```python
from build123d import *

# Parameters (mm, degrees)
F0_R     = 12.5
F1_DEPTH = 3.175
F3_DEPTH = 25.4
F4_R     = 1.5
F5_DEPTH = 25


with BuildPart() as f1:
    # F0 (on Top) → F1 (new body)
    with BuildSketch(Plane.XY):
        with BuildLine():
            Line((61, 42.8), (-61, 42.8))
            ThreePointArc((-61, 42.8), (-63.12132, 41.92132), (-64, 39.8))
            Line((-64, 39.8), (-64, -39.8))
            ThreePointArc((-64, -39.8), (-63.12132, -41.92132), (-61, -42.8))
            Line((-61, -42.8), (61, -42.8))
            ThreePointArc((61, -42.8), (63.12132, -41.92132), (64, -39.8))
            Line((64, -39.8), (64, 39.8))
            ThreePointArc((64, 39.8), (63.12132, 41.92132), (61, 42.8))
        make_face()
        Circle(F0_R, mode=Mode.SUBTRACT)
    extrude(amount=F1_DEPTH)

    # F2 (on Top) → F3 (join)
    with BuildSketch(Plane.XY):
        with BuildLine():
            Line((-57.674601, -36.461943), (-64.024601, -36.461943))
            Line((-64.024601, -36.461943), (-64.024601, -39.811943))
            ThreePointArc((-64.024601, -39.811943), (-63.145921, -41.933263), (-61.024601, -42.811943))
            Line((-61.024601, -42.811943), (-57.674601, -42.811943))
            Line((-57.674601, -42.811943), (-57.674601, -36.461943))
        make_face()
    extrude(amount=-F3_DEPTH)

    # F4 (on Top) → F5 (cut)
    with BuildSketch(Plane.XY):
        with Locations((-48.248243, 0)):
            Circle(F4_R)
        with Locations((48.708693, 0)):
            Circle(F4_R)
    extrude(amount=F5_DEPTH, mode=Mode.SUBTRACT)


solid = f1.part
```
Geometry check sheet. Reference: the model listing, model coordinates, mm. A direction names the side the tool comes from. Coordinates: 2 decimals unless noted, no trailing zeros. Loops run counter-clockwise (first coordinate to the right, second up) from the corner with the lowest first, then second, coordinate; pieces in that order, holes last. Notation, with made-up numbers: (80, 68.5) -> (128, 68.5) arc R17 cw to (128, 82.5) -> close; hole circle Ø4 at (33, 50.5). An arc over 180 degrees is marked (long way). Put each result on its own line as item: value.
1) Cross-section at D-D on x = 56.5. Record the boundary of the cut face in (y, z) (3 decimals), plus the area to 3 significant figures.
Result set:
outline: (-42.8, 0) -> (42.8, 0) -> (42.8, 3.175) -> (-42.8, 3.175) -> close
area: 272 mm^2
2) Release check for a two-part mould opening along Y. For faces 1 (the cylindrical face through (-49.747, 0.066, 1.565)), 2 (the flat face through (64, -1, 2)), 3 (the cylindrical face through (-63.17, -41.91, -12.52)), 4 (the flat face through (1, 42.8, 2)) record: released by +Y, released by -Y, zero draft, split by the parting line, or undercut.
Result set:
face 1: undercut
face 2: zero draft
face 3: released by -Y
face 4: released by +Y
3) Tool access check on faces 5 (the flat face through (-57.675, -40, -13)), 6 (the flat face through (-59, -42.812, -13)), 7 (the flat face through (-61, -36.462, -13)). Record the directions out of +Z, -Z, +X, -X, +Y, -Y that give a thin tool (end or side, any length) a straight path to the whole face; none if there is none.
Result set:
face 5: -Z, +X, +Y, -Y
face 6: +Z, -Z, +X, -X, -Y
face 7: -Z, +X, -X, +Y
4) Cross-section at B-B on x = 0. Record the boundary of the cut face in (y, z) (3 decimals).
Result set:
outline: (-42.8, 0) -> (-12.5, 0) -> (-12.5, 3.175) -> (-42.8, 3.175) -> close; (12.5, 0) -> (42.8, 0) -> (42.8, 3.175) -> (12.5, 3.175) -> close
5) Cross-section at A-A on y = 0. Record the boundary of the cut face in (x, z) (3 decimals), plus the area to 3 significant figures.
Result set:
outline: (-64, 0) -> (-49.748, 0) -> (-49.748, 3.175) -> (-64, 3.175) -> close; (-46.748, 0) -> (-12.5, 0) -> (-12.5, 3.175) -> (-46.748, 3.175) -> close; (12.5, 0) -> (47.209, 0) -> (47.209, 3.175) -> (12.5, 3.175) -> close; (50.209, 0) -> (64, 0) -> (64, 3.175) -> (50.209, 3.175) -> close
area: 308 mm^2
6) Thickness scan on line 1 (Y direction, x = 0, z = 0.7); line 2 (Z direction, x = 17, y = -3) (3 decimals); line 3 (Y direction, x = -58.5, z = -20.75). Record the ranges inside material, lowest first.
Result set:
line 1: y = -42.8 to -12.5, 12.5 to 42.8
line 2: z = 0 to 3.175
line 3: y = -42.81 to -36.46
7) Cross-section at C-C on z = -13.75. Record the boundary of the cut face in (x, y), plus the area to 3 significant figures.
Result set:
outline: (-64.02, -39.81) arc R3 ccw to (-61.02, -42.81) -> (-57.67, -42.81) -> (-57.67, -36.46) -> (-64.02, -36.46) -> close
area: 38.4 mm^2
8) Gauge pin test, flat ends, axial feed: pin 1 Ø1 at (y, z) = (10.5, 2.5) entering from -X; pin 2 Ø1.8 at (x, y) = (-48.25, 0) entering from -Z; pin 3 Ø2.5 at (x, z) = (30, 2) entering from -Y; pin 4 Ø1.9 at (y, z) = (-39, -16.5) entering from +X. Record the tip position at first contact, or that the pin passes through.
Result set:
pin 1: stops at x = -64
pin 2: passes through
pin 3: stops at y = -42.8
pin 4: stops at x = -57.67
